Could you check a few things on this model? Use its own coordinates, in mm. Coordinates: 2 decimals unless noted, no trailing zeros. Order: outer loops, then holes, each group sorted by start corner. A loop starts at its lowest first (then second) coordinate and runs counter-clockwise, first axis right, second up. Notation, with made-up numbers: (45.25, -16.75) - (62.25, -16.75) arc R16 cw to (62.25, 5.25) - close; hole circle Ø7 at (56, -25). An arc over 180 degrees is marked (long way). One line per item, written item: value.
Autodesk Inventor part; units mm, degrees
ref_plane "Start Plane" through (0, 0, 20) normal (0, 0, 1) x (1, 0, 0)
ref_plane "End Plane" through (0, 0, 1330) normal (0, 0, 1) x (1, 0, 0)
ref_plane "Work Plane4" through (0, -984.5, 1330) normal (0, 0, 1) x (1, 0, 0)
ref_plane "Start Plane" through (0, 0, 20) normal (0, 0, 1) x (1, 0, 0)
ref_plane "End Plane" through (0, 0, 1330) normal (0, 0, 1) x (1, 0, 0)
sketch "Sketch" plane through (0, 0, 0) normal (0, 0, 1) x (1, 0, 0)
  line L0 (-20, -15.5) -> (-20, 15.5)
  line L1 (-15.5, 20) -> (15.5, 20)
  line L2 (20, 15.5) -> (20, -15.5)
  line L3 (15.5, -20) -> (-15.5, -20)
  arc A0 (-20, -15.5) -> (-15.5, -20) centre (-15.5, -15.5) ccw
  arc A1 (-15.5, 20) -> (-20, 15.5) centre (-15.5, 15.5) ccw
  arc A2 (20, 15.5) -> (15.5, 20) centre (15.5, 15.5) ccw
  arc A3 (15.5, -20) -> (20, -15.5) centre (15.5, -15.5) ccw
  arc A4 (-15.5, 17) -> (-17, 15.5) centre (-15.5, 15.5) ccw
  line L4 (-15.5, 17) -> (15.5, 17)
  arc A5 (17, 15.5) -> (15.5, 17) centre (15.5, 15.5) ccw
  line L5 (17, 15.5) -> (17, -15.5)
  arc A6 (15.5, -17) -> (17, -15.5) centre (15.5, -15.5) ccw
  line L6 (15.5, -17) -> (-15.5, -17)
  arc A7 (-17, -15.5) -> (-15.5, -17) centre (-15.5, -15.5) ccw
  line L7 (-17, -15.5) -> (-17, 15.5)
  line L8 (0, 29.3048) -> (0, -29.3048) construction
  line L9 (-29.3048, 0) -> (29.3048, 0) construction
  dimension "d7" = 4.5
  dimension "d10" = 40
  dimension "d11" = 40
  dimension "d12" = 3
  dimension "d15" = 20
  dimension "d16" = 20
extrude "Body" add sketch "Sketch" along normal up to surface (1310 mm away) from surface at 20
sketch "Sketch3" plane through (0, 0, 0) normal (0, 0, 1) x (1, 0, 0)
  line L0 (0, 0) -> (10, 0)
ref_plane "Work Plane3" through (0, 0, 0) normal (0, -1, 0) x (1, 0, 0)
ref_plane "Work Plane4" through (0, -984.5, 1330) normal (0, 0, 1) x (1, 0, 0)
split "Split1" plane through (0, -984.5, 1330) removes the side toward (0, 0, 1)
ref_plane "Work Plane5" through (0, -15.5, 20) normal (0, 0, -1) x (-1, 0, 0)
split "Split2" plane through (0, -15.5, 20) removes the side toward (0, 0, -1)
sketch "Sketch4" plane through (0, 0, 0) normal (0, -1, 0) x (1, 0, 0)
  line L0 (-2, 20) -> (12, 20)
  line L1 (-2, 1330) -> (12, 1330)
  dimension "d18" = 1310
equation "\"d7\" = G_IR"
equation "\"d10\" = G_H"
equation "\"d11\" = G_W"
equation "\"d12\" = G_T"
equation "\"d15\" = 0.5 * d10"
equation "\"d16\" = 0.5 * d11"
equation "\"d3\" = G_L"
equation "\"G_W\" = 40"
equation "\"G_H\" = 40"
equation "\"G_T\" = 3"
equation "\"G_IR\" = 4.5"
equation "\"G_L\" = d18"
properties part number "ISO 12633-2 - 40x40x3 - 1310" material "Steel, Mild"
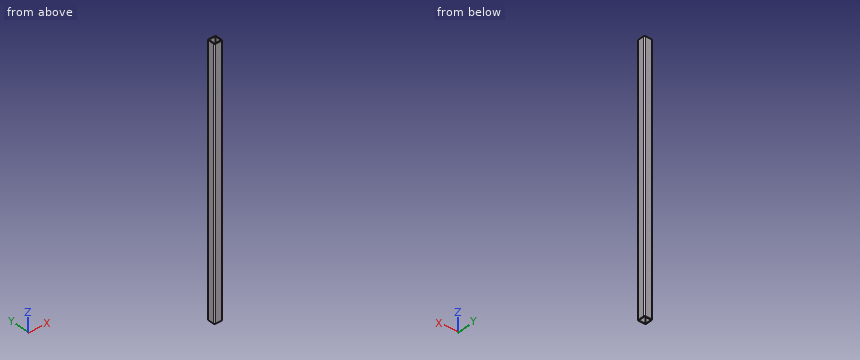
Item 1: I want a section at A-A on y = 2. Please give me the cut outline in (x, z), then the cut area to 3 significant figures.
Conclusion:
outline: (-20, 20) - (-17, 20) - (-17, 1330) - (-20, 1330) - close; (17, 20) - (20, 20) - (20, 1330) - (17, 1330) - close
area: 7,860 mm²
Item 2: I want a section at C-C on z = 682.5. Please give me the cut outline in (x, y), then the cut area to 3 significant figures.
Conclusion:
outline: (-20, -15.5) arc R4.5 ccw to (-15.5, -20) - (15.5, -20) arc R4.5 ccw to (20, -15.5) - (20, 15.5) arc R4.5 ccw to (15.5, 20) - (-15.5, 20) arc R4.5 ccw to (-20, 15.5) - close; hole (-17, -15.5) arc R1.5 ccw to (-15.5, -17) - (15.5, -17) arc R1.5 ccw to (17, -15.5) - (17, 15.5) arc R1.5 ccw to (15.5, 17) - (-15.5, 17) arc R1.5 ccw to (-17, 15.5) - close
area: 429 mm²
Item 3: If I drill on probe 1 along X at (y, z) = (-13, 179); probe 2 along Y at (x, z) = (16, 979), over which ranges is the centre line in solid material (lowest first)?
Conclusion:
probe 1: -20 to -17, 17 to 20
probe 2: -19.97 to -16.91, 16.91 to 19.97
